Can you work these out from the model? Positions are in its coordinate system, mm. Give positions to 0.01 mm unless a question says otherwise; leave off trailing zeros. Write each loop counter-clockwise with the first axis right and the second up, starting at its lowest first coordinate (ties: lowest second). Pieces come first, ordered by that corner, then holes.
1. I'm going to push flat-ended pins straight in: pin 1 (0.6 mm diameter, centred on y = -1160, z = 49.5, fed in from +X); pin 2 (0.8 mm diameter, centred on x = 750, z = 41.5, fed in from -Y); pin 3 (0.5 mm diameter, centred on y = -538.5, z = 41.5, fed in from +X); pin 4 (2 mm diameter, centred on y = -716.5, z = 44.5, fed in from +X). Where does each tip first touch, or does it pass through?
2. Suppose I cut it at B-B (z = 47.25). Please give me the cut outline in (x, y), and give its area (3 significant figures).
3. If I drill on probe 1 along Z at (x, y) = (1161, -735); probe 2 along Y at (x, z) = (1088, 41.5), over which ranges is the centre line in solid material (lowest first)?
4. Suppose I cut it at A-A (x = 896). Please give me the cut outline in (y, z), and give its area (3 significant figures).
5. Suppose I cut it at D-D (y = -1019.5). Please give me the cut outline in (x, z), and give its area (3 significant figures).
6. Suppose I cut it at C-C (x = 969). Please give me the cut outline in (y, z), and give its area (3 significant figures).
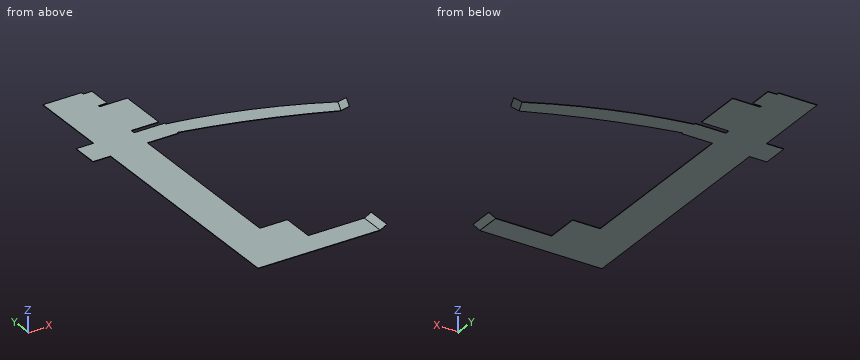
```python
from build123d import *

# Parameters (mm, degrees)
SKETCH_1_W      = 19
SKETCH_1_H      = 52
SKETCH_1_W_2    = 60
SKETCH_1_H_2    = 29.5
SKETCH_1_H_3    = 41.5
SKETCH_1_H_4    = 49.5
SKETCH_1_H_5    = 60
SKETCH_1_H_6    = 106.4
SKETCH_1_H_7    = 111
SKETCH_1_H_8    = 112
SKETCH_1_H_9    = 113
SKETCH_1_H_10   = 116.5
EXTRUDE_1_DEPTH = 1
EXTRUDE_2_DEPTH = 53.5
EXTRUDE_3_DEPTH = 33.4


with BuildPart() as part:
    # 草图1 → 拉伸1 (new body)
    with BuildSketch(Plane.XY.offset(42)):
        with Locations((858.7, -476.2)):
            Rectangle(SKETCH_1_W, SKETCH_1_H)
        with Locations((879.2, -1106.35)):
            Rectangle(SKETCH_1_W_2, SKETCH_1_H_2)
        with Locations((879.2, -1070.85)):
            Rectangle(SKETCH_1_W_2, SKETCH_1_H_3)
        with Locations((795.5, -1149.85)):
            Rectangle(SKETCH_1_W_2, SKETCH_1_H_4)
        with Locations((795.5, -474.2)):
            Rectangle(SKETCH_1_W_2, SKETCH_1_H_5)
        with Locations((879.2, -559.9)):
            Rectangle(SKETCH_1_W_2, SKETCH_1_H_6)
        with Locations((795.5, -953.1)):
            Rectangle(SKETCH_1_W_2, SKETCH_1_H_7)
        with Locations((795.5, -842.1)):
            Rectangle(SKETCH_1_W_2, SKETCH_1_H_7)
        with Locations((795.5, -560.2)):
            Rectangle(SKETCH_1_W_2, SKETCH_1_H_8)
        with Locations((795.5, -730.1)):
            Rectangle(SKETCH_1_W_2, SKETCH_1_H_9)
        with Locations((795.5, -1066.85)):
            Rectangle(SKETCH_1_W_2, SKETCH_1_H_10)
        Polygon((1031.2, -1174.6), (1031.2, -1121.1), (909.2, -1121.1), (849.2, -1121.1), (849.2, -1174.6), align=None)
        with BuildLine():
            Line((1213.4, -757.7), (1226.4, -727))
            ThreePointArc((1226.4, -727), (1075.34720829, -664.295577574), (916.2, -626.6))
            Line((916.2, -626.6), (916.2, -623.1))
            Line((916.2, -623.1), (849.2, -623.1))
            Line((849.2, -623.1), (849.2, -668.1))
            Line((849.2, -668.1), (916.2, -668.1))
            Line((916.2, -668.1), (916.2, -664.6))
            ThreePointArc((916.2, -664.6), (1067.153405165, -703.637303814), (1213.4, -757.7))
        make_face()
        Polygon((849.2, -450.2), (849.2, -444.2), (825.5, -444.2), (825.5, -504.2), (825.5, -616.2), (765.5, -616.2), (727.5, -616.2), (727.5, -673.6), (765.5, -673.6), (825.5, -673.6), (825.5, -786.6), (825.5, -897.6), (825.5, -1008.6), (825.5, -1125.1), (825.5, -1174.6), (849.2, -1174.6), (849.2, -1121.1), (849.2, -1091.6), (849.2, -1050.1), (849.2, -681.1), (849.2, -668.1), (849.2, -623.1), (849.2, -613.1), (849.2, -506.7), (849.2, -502.2), align=None)
    extrude(amount=-EXTRUDE_1_DEPTH)

    # 草图2 → 拉伸2 (add)
    with BuildSketch(Plane.XZ.offset(1174.6)):
        Polygon((1031.2, 42), (1046.2, 49.648642972), (1046.2, 49.148642972), (1031.2, 41.5), align=None)
    extrude(amount=-EXTRUDE_2_DEPTH)

    # 草图3 → 拉伸3 (add)
    with BuildSketch(Plane(origin=(1226.4, -727, 42), x_dir=(-0.9208430096491422, 0.38993352200126363, 0), z_dir=(0.38993352200126363, 0.9208430096491422, 0))):
        Polygon((0, -0.5), (-15.5, 7.15), (-15.5, 7.65), (0, 0), align=None)
    extrude(amount=-EXTRUDE_3_DEPTH)


solid = part.part
```
Checks:
1. pin 1: stops at x = 1046.2
1. pin 2: stops at y = -673.6
1. pin 3: stops at x = 909.2
1. pin 4: passes through
2. outline: (1041.5, -1174.6) - (1042.48, -1174.6) - (1042.48, -1121.1) - (1041.5, -1121.1) - close; (1223.17, -761.9) - (1224.1, -762.3) - (1237.13, -731.54) - (1236.2, -731.15) - close
2. area: 86.3 mm2
3. probe 1: z = 41 to 42
3. probe 2: y = -710.33 to -668.48
4. outline: (-1174.6, 41) - (-1050.1, 41) - (-1050.1, 42) - (-1174.6, 42) - close; (-668.1, 41) - (-623.1, 41) - (-623.1, 42) - (-668.1, 42) - close; (-613.1, 41) - (-506.7, 41) - (-506.7, 42) - (-613.1, 42) - close
4. area: 276 mm2
5. outline: (765.5, 41) - (849.2, 41) - (849.2, 42) - (765.5, 42) - close
5. area: 83.7 mm2
6. outline: (-1174.6, 41) - (-1121.1, 41) - (-1121.1, 42) - (-1174.6, 42) - close; (-676.41, 41) - (-636.13, 41) - (-636.13, 42) - (-676.41, 42) - close
6. area: 93.8 mm2
